```python
from build123d import *

# Parameters (mm, degrees)
SKETCH2_R           = 1
BOSS_EXTRUDE1_DEPTH = 7
CUT_EXTRUDE1_START  = -5
SKETCH3_R           = 1.15
CUT_EXTRUDE1_DEPTH  = 13
SKETCH5_R           = 2.5
CUT_EXTRUDE2_DEPTH  = 2
CUT_EXTRUDE3_START  = 7
SKETCH5_2_R         = 2.5
CUT_EXTRUDE3_DEPTH  = 2
BOSS_EXTRUDE2_START = -5
BOSS_EXTRUDE2_DEPTH = 13
CUT_EXTRUDE4_START  = 17.4
SKETCH7_W           = 12
SKETCH7_H           = 6
CUT_EXTRUDE4_DEPTH  = 6
CUT_EXTRUDE5_START  = 17.4
SKETCH8_W           = 15
SKETCH8_H           = 13
CUT_EXTRUDE5_DEPTH  = 1.6
CUT_EXTRUDE6_START  = 15.8
SKETCH9_W           = 13
SKETCH9_H           = 3
CUT_EXTRUDE6_DEPTH  = 1
BOSS_EXTRUDE3_START = 8
SKETCH10_W          = 5.4
SKETCH10_H          = 5
BOSS_EXTRUDE3_DEPTH = 13
CUT_EXTRUDE7_START  = 8
SKETCH11_W          = 17.4
SKETCH11_H          = 3
CUT_EXTRUDE7_DEPTH  = 13
BOSS_EXTRUDE4_START = 15
SKETCH12_W          = 3
SKETCH12_H          = 4
BOSS_EXTRUDE4_DEPTH = 3
CUT_EXTRUDE8_START  = 8
SKETCH13_W          = 3.2
SKETCH13_H          = 5.2
CUT_EXTRUDE8_DEPTH  = 3.2


with BuildPart() as part:
    # Sketch2 → Boss-Extrude1 (new body)
    with BuildSketch(Plane(origin=(0, 0, 0), x_dir=(0, 0, -1), z_dir=(1, 0, 0))):
        with BuildLine():
            Line((3.494281042, -5), (15, -5))
            Line((15, -5), (15, 8))
            Line((15, 8), (-15, 8))
            Line((-15, 8), (-15, -5))
            Line((-15, -5), (-3.494281042, -5))
            ThreePointArc((-3.494281042, -5), (-4.313351365, -4.313351365), (-5, -3.494281042))
            Line((-5, -3.494281042), (-5, 3.494281042))
            ThreePointArc((-5, 3.494281042), (0, 6.1), (5, 3.494281042))
            Line((5, 3.494281042), (5, -3.494281042))
            ThreePointArc((5, -3.494281042), (4.313351365, -4.313351365), (3.494281042, -5))
        make_face()
        with Locations((-11.25, 0)):
            Circle(SKETCH2_R, mode=Mode.SUBTRACT)
        with Locations((11.25, 0)):
            Circle(SKETCH2_R, mode=Mode.SUBTRACT)
    extrude(amount=BOSS_EXTRUDE1_DEPTH)

    # Sketch3 → Cut-Extrude1 (cut)
    with BuildSketch(Plane(origin=(0, 0, 0), x_dir=(1, 0, 0), z_dir=(0, 1, 0)).offset(CUT_EXTRUDE1_START)):
        with Locations((3.5, 8.494281042)):
            Circle(SKETCH3_R)
        with Locations((3.5, -8.494281042)):
            Circle(SKETCH3_R)
    extrude(amount=CUT_EXTRUDE1_DEPTH, mode=Mode.SUBTRACT)

    # Sketch5 → Cut-Extrude2 (cut)
    with BuildSketch(Plane(origin=(0, 0, 0), x_dir=(0, 0, -1), z_dir=(1, 0, 0))):
        with Locations((11.25, 0)):
            Circle(SKETCH5_R)
        with Locations((-11.25, 0)):
            Circle(SKETCH5_R)
    extrude(amount=CUT_EXTRUDE2_DEPTH, mode=Mode.SUBTRACT)

    # Sketch5<2> → Cut-Extrude3 (cut)
    with BuildSketch(Plane(origin=(0, 0, 0), x_dir=(0, 0, -1), z_dir=(1, 0, 0)).offset(CUT_EXTRUDE3_START)):
        with Locations((11.25, 0)):
            Circle(SKETCH5_2_R)
        with Locations((-11.25, 0)):
            Circle(SKETCH5_2_R)
    extrude(amount=-CUT_EXTRUDE3_DEPTH, mode=Mode.SUBTRACT)

    # Sketch6 → Boss-Extrude2 (add)
    with BuildSketch(Plane(origin=(0, 0, 0), x_dir=(1, 0, 0), z_dir=(0, 1, 0)).offset(BOSS_EXTRUDE2_START)):
        Polygon((0, 15), (7, 15), (7, 22), (12.4, 22), (12.4, 5), (17.4, 5), (17.4, 25), (0, 25), align=None)
    extrude(amount=BOSS_EXTRUDE2_DEPTH)

    # Sketch7 → Cut-Extrude4 (cut)
    with BuildSketch(Plane(origin=(0, 0, 0), x_dir=(0, 0, -1), z_dir=(1, 0, 0)).offset(CUT_EXTRUDE4_START)):
        with Locations((11, 0)):
            Rectangle(SKETCH7_W, SKETCH7_H)
    extrude(amount=-CUT_EXTRUDE4_DEPTH, mode=Mode.SUBTRACT)

    # Sketch8 → Cut-Extrude5 (cut)
    with BuildSketch(Plane(origin=(0, 0, 0), x_dir=(0, 0, -1), z_dir=(1, 0, 0)).offset(CUT_EXTRUDE5_START)):
        with Locations((12.5, 1.5)):
            Rectangle(SKETCH8_W, SKETCH8_H)
    extrude(amount=-CUT_EXTRUDE5_DEPTH, mode=Mode.SUBTRACT)

    # Sketch9 → Cut-Extrude6 (cut)
    with BuildSketch(Plane(origin=(0, 0, 0), x_dir=(0, 0, -1), z_dir=(1, 0, 0)).offset(CUT_EXTRUDE6_START)):
        with Locations((11.5, 6.5)):
            Rectangle(SKETCH9_W, SKETCH9_H)
    extrude(amount=-CUT_EXTRUDE6_DEPTH, mode=Mode.SUBTRACT)

    # Sketch10 → Boss-Extrude3 (add)
    with BuildSketch(Plane(origin=(0, 0, 0), x_dir=(1, 0, 0), z_dir=(0, 1, 0)).offset(BOSS_EXTRUDE3_START)):
        with Locations((9.7, 19.5)):
            Rectangle(SKETCH10_W, SKETCH10_H)
    extrude(amount=-BOSS_EXTRUDE3_DEPTH)

    # Sketch11 → Cut-Extrude7 (cut)
    with BuildSketch(Plane(origin=(0, 0, 0), x_dir=(1, 0, 0), z_dir=(0, 1, 0)).offset(CUT_EXTRUDE7_START)):
        with Locations((8.7, 23.5)):
            Rectangle(SKETCH11_W, SKETCH11_H)
    extrude(amount=-CUT_EXTRUDE7_DEPTH, mode=Mode.SUBTRACT)

    # Sketch12 → Boss-Extrude4 (add)
    with BuildSketch(Plane.XY.offset(BOSS_EXTRUDE4_START)):
        with Locations((3.5, 3)):
            Rectangle(SKETCH12_W, SKETCH12_H)
    extrude(amount=BOSS_EXTRUDE4_DEPTH)

    # Sketch13 → Cut-Extrude8 (cut)
    with BuildSketch(Plane(origin=(0, 0, 0), x_dir=(1, 0, 0), z_dir=(0, 1, 0)).offset(CUT_EXTRUDE8_START)):
        with Locations((3.5, 14.5)):
            Rectangle(SKETCH13_W, SKETCH13_H)
    extrude(amount=-CUT_EXTRUDE8_DEPTH, mode=Mode.SUBTRACT)


solid = part.part
```
The model under review builds one solid part; all positions refer to its coordinate system, in mm. A direction names the side the tool comes from. Round coordinates to 2 decimals unless told otherwise and drop trailing zeros. Loops run counter-clockwise (first coordinate to the right, second up) from the corner with the lowest first, then second, coordinate; pieces in that order, holes last. Notation, with made-up numbers: M -39.75,-22 L -5.75,-22 A31 cw -5.75,17 Z; hole C 43.25,62.5 d2. An arc over 180 degrees is marked long. Answer as a JSON object with one key per item and string values.
(1) Take a section at A-A on x = 3.5. Give the boundary of the cut face in (y, z).
Resolved:
{"outline": "M -5,-22 L 8,-22 L 8,-17.1 L 4.8,-17.1 L 4.8,-11.9 L 8,-11.9 L 8,-9.64 L -5,-9.64 Z; M -5,-7.34 L 8,-7.34 L 8,7.34 L -5,7.34 L -5,3.49 A6.1 cw -3.49,5 L 3.49,5 A6.1 cw 3.49,-5 L -3.49,-5 A6.1 cw -5,-3.49 Z; M -5,9.64 L 8,9.64 L 8,15 L 5,15 L 5,18 L 1,18 L 1,15 L -5,15 Z; hole C 0,-11.25 d2; hole C 0,11.25 d2"}
(2) Take a section at B-B on z = -6. Give the boundary of the cut face in (x, y), and give its area (3 significant figures).
Resolved:
{"outline": "M 0,-5 L 7,-5 L 7,8 L 0,8 Z; M 12.4,-5 L 15.8,-5 L 15.8,-3 L 12.4,-3 Z; M 12.4,3 L 15.8,3 L 15.8,5 L 14.8,5 L 14.8,8 L 12.4,8 Z", "area": "112 mm²"}
(3) Tool access review of faces 4 (the flat face through (5, 0, 10)), 5 (the flat face through (5.1, 6, -14)), 6 (the flat face through (14, -4, -5)), 7 (the flat face through (3, 5, 16)), 8 (the flat face through (2, 3, 16)): name each direction out of +Z, -Z, +X, -X, +Y, -Y from which nothing blocks a thin tool from reaching the whole face with its end or side.
Resolved:
{"face 4": "+X", "face 5": "+Y", "face 6": "+Z, +X, +Y, -Y", "face 7": "+Z, +X, -X, +Y", "face 8": "+Z, -X, +Y, -Y"}
(4) To check wall thickness, follow line 1 along Z through (x, y) = (3.5, -1.5); line 2 along X through (y, z) = (6, -7); line 3 along Z through (x, y) = (4.25, 0). State the ranges of each line that lie inside material, in increasing order.
Resolved:
{"line 1": "-22 to -9.64, -7.34 to -5, 5 to 7.34, 9.64 to 15", "line 2": "0 to 7, 12.4 to 14.8", "line 3": "-22 to -12.25, -10.25 to -9.37, -7.62 to -5, 5 to 7.62, 9.37 to 10.25, 12.25 to 15"}
(5) Take a section at C-C on y = -2. Count the separate pieces of the cut face and the enclosed holes in it, and give its area (3 significant figures).
Resolved:
{"separate pieces": "2", "enclosed holes": "2", "area": "204 mm²"}
(6) Clearance check with flat-ended pins moving along their axes: P1, Ø2.5, axis at x = 4, y = 6.5, coming from the +Z side; P2, Ø1.5, axis at y = 5, z = -10, coming from the -X side; P3, Ø2.5, axis at x = 12.5, y = 0.5, coming from the +Z side; P4, Ø2.5, axis at y = 0, z = 11.25, coming from the +X side. State where each tip first meets the part, or that it passes through.
Resolved:
{"P1": "z = 15", "P2": "x = 0", "P3": "z = -17", "P4": "x = 5"}
(7) Draft analysis for pull direction Z (two halves, no side actions). For faces 1 (the flat face through (5, 3, 16)), 2 (the flat face through (3, 0, 5)), 3 (the flat face through (15, 6, -18)), state which applies: released by +Z, released by -Z, zero draft, split by the parting line, or undercut.
Resolved:
{"face 1": "zero draft", "face 2": "undercut", "face 3": "released by +Z"}
(8) Take a section at D-D on y = 5.5. Give the boundary of the cut face in (x, z).
Resolved:
{"outline": "M 0,-22 L 17.4,-22 L 17.4,-20 L 15.8,-20 L 15.8,-18 L 14.8,-18 L 14.8,-5 L 12.4,-5 L 12.4,-17 L 7,-17 L 7,-2.64 L 0,-2.64 Z; M 0,2.64 L 7,2.64 L 7,15 L 0,15 Z; hole M 1.9,-17.1 L 5.1,-17.1 L 5.1,-11.9 L 1.9,-11.9 Z; hole C 3.5,-8.49 d2.3; hole C 3.5,8.49 d2.3"}
